Check sheet for the modelled part. Datum: model origin and axes. Units: mm. A direction names the side the tool comes from. Give positions to 0.01 mm unless a question says otherwise; leave off trailing zeros. Loops run counter-clockwise (first coordinate to the right, second up) from the corner with the lowest first, then second, coordinate; pieces in that order, holes last. Notation, with made-up numbers: (11, -5) - (25, -5) arc R15 cw to (25, 4) - close; hole circle Ø4 at (19.25, 4). An arc over 180 degrees is marked (long way). Use CSV: the item, a comma, the result in double quotes.
from build123d import *

# Parameters (mm, degrees)
SKETCH_1_R           = 19.25
SKETCH_1_R_2         = 16.25
EXTRUDE_1_DEPTH      = 1
SKETCH_3_R           = 20.25
SKETCH_3_R_2         = 19.25
SKETCH_3_R_3         = 16.25
SKETCH_3_R_4         = 15.25
EXTRUDE_3_DEPTH      = 10
EXTRUDE_3_DEPTH_BACK = 1


with BuildPart() as part:
    # 草图1 → 凸台-拉伸1 (new body)
    with BuildSketch(Plane(origin=(0, 0, 0), x_dir=(1, 0, 0), z_dir=(0, 1, 0))):
        Circle(SKETCH_1_R)
        Circle(SKETCH_1_R_2, mode=Mode.SUBTRACT)
    extrude(amount=EXTRUDE_1_DEPTH)

    # 草图3 → 凸台-拉伸3 (add, two sides)
    with BuildSketch(Plane(origin=(0, 1, 0), x_dir=(1, 0, 0), z_dir=(0, 1, 0))) as extrude_3_sk:
        Circle(SKETCH_3_R)
        Circle(SKETCH_3_R_2, mode=Mode.SUBTRACT)
        Circle(SKETCH_3_R_3)
        Circle(SKETCH_3_R_4, mode=Mode.SUBTRACT)
    extrude(amount=EXTRUDE_3_DEPTH)
    extrude(extrude_3_sk.sketch, amount=-EXTRUDE_3_DEPTH_BACK)


solid = part.part
1. Sectioned sample at B-B, the plane x = 0. Record the boundary of the cut face in (y, z), and give its area (3 significant figures).
Completed:
outline,"(0, -20.25) - (11, -20.25) - (11, -19.25) - (1, -19.25) - (1, -16.25) - (11, -16.25) - (11, -15.25) - (0, -15.25) - close; (0, 15.25) - (11, 15.25) - (11, 16.25) - (1, 16.25) - (1, 19.25) - (11, 19.25) - (11, 20.25) - (0, 20.25) - close"
area,"50.0 mm²"
2. Go/stop test with flat-tipped pins: pin 1 Ø5 at (x, y) = (12, 9.5) entering from +Z; pin 2 Ø3 at (x, z) = (-11, 5) entering from -Y; pin 3 Ø4 at (y, z) = (2.5, -10.5) entering from +X; pin 4 Ø1 at (x, y) = (-15, 5) entering from +Z. Record where each tip stops, or that it passes through.
Completed:
pin 1,"stops at z = 17.88"
pin 2,"passes through"
pin 3,"stops at x = 18.38"
pin 4,"stops at z = 14.14"
3. Sectioned sample at A-A, the plane z = 0. Record the boundary of the cut face in (x, y).
Completed:
outline,"(-20.25, 0) - (-15.25, 0) - (-15.25, 11) - (-16.25, 11) - (-16.25, 1) - (-19.25, 1) - (-19.25, 11) - (-20.25, 11) - close; (15.25, 0) - (20.25, 0) - (20.25, 11) - (19.25, 11) - (19.25, 1) - (16.25, 1) - (16.25, 11) - (15.25, 11) - close"
4. Scan lines: line 1 along X through (y, z) = (8.75, 0); line 2 along Z through (x, y) = (0.5, 6.5); line 3 along Z through (x, y) = (-9, 7). Record each from-to range of solid material in increasing order.
Completed:
line 1,"x = -20.25 to -19.25, -16.25 to -15.25, 15.25 to 16.25, 19.25 to 20.25"
line 2,"z = -20.24 to -19.24, -16.24 to -15.24, 15.24 to 16.24, 19.24 to 20.24"
line 3,"z = -18.14 to -17.02, -13.53 to -12.31, 12.31 to 13.53, 17.02 to 18.14"
5. Set-up check for faces 1 (the face through (7, 0, -14)), 2 (the face through (15.5, 5.93, -4.88)): record each of +Z, -Z, +X, -X, +Y, -Y from which the full face is reachable in a straight line by a thin tool's end or side.
Completed:
face 1,"+Z, -Z, +X, -X, -Y"
face 2,"+Y"
6. Release check for a two-part mould opening along Z. For faces 3 (the face through (-13, 1, 10)), 4 (the face through (11, 6, -17)), 5 (the face through (10.4, 11, 16.4)) record: released by +Z, released by -Z, zero draft, split by the parting line, or undercut.
Completed:
face 3,"undercut"
face 4,"split by the parting line"
face 5,"zero draft"
7. Sectioned sample at C-C, the plane y = 9.25. Record the boundary of the cut face in (x, z).
Completed:
outline,"circle Ø40.5 at (0, 0); circle Ø32.5 at (0, 0); hole circle Ø38.5 at (0, 0); hole circle Ø30.5 at (0, 0)"
